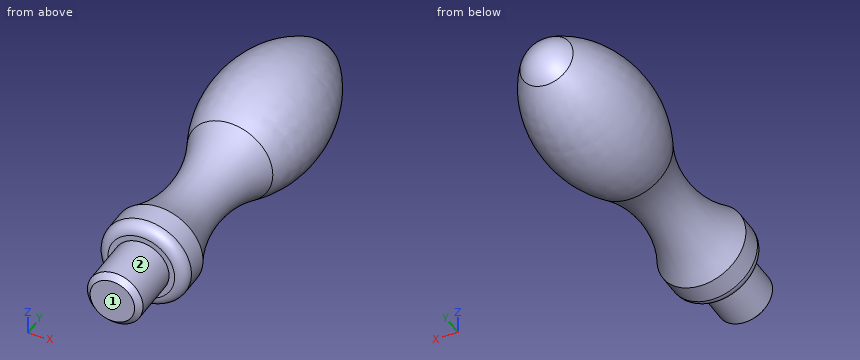
from build123d import *


with BuildPart() as part:
    # Sketch1 → Revolve1 (revolve)
    with BuildSketch(Plane.XY):
        with BuildLine():
            Line((0, 0), (4, 0))
            Line((4, 0), (5, 1))
            Line((5, 1), (5, 10))
            Line((5, 10), (6, 10))
            ThreePointArc((6, 10), (7.414213562, 10.585786438), (8, 12))
            Line((8, 12), (8, 16))
            ThreePointArc((8, 16), (5, 28.303061069), (7.726981853, 40.669502823))
            ThreePointArc((7.726981853, 40.669502823), (10.3121962, 55.557059673), (4.784815021, 69.620158175))
            ThreePointArc((4.784815021, 69.620158175), (2.671989048, 71.372194573), (0, 72))
            Line((0, 72), (0, 0))
        make_face()
    revolve(axis=Axis((0, -4.536906655, 0), (0, 1, 0)))


solid = part.part
Input: part model. Units: mm. Frame: model coordinates. Face numbers are marked on the shaded views. A direction names the side the tool comes from. Round coordinates to 2 decimals unless told otherwise and drop trailing zeros. Loops run counter-clockwise (first coordinate to the right, second up) from the corner with the lowest first, then second, coordinate; pieces in that order, holes last. Notation, with made-up numbers: M -35.5,-20.75 L -24.5,-20.75 A26 cw -24.5,-4.75 Z; hole C 28.25,27.5 d7. An arc over 180 degrees is marked long. Answer as CSV lines item,"result". Start each with the question number.
(1) Reachability of the marked faces 1 and 2 from +Z, -Z, +X, -X, +Y, -Y: full face, straight path, thin tool, end or side. Return the list, or none.
(2) Line query: line 1 (X direction, y = 11, z = 5.25); line 2 (X direction, y = 58, z = 4.75); line 3 (Z direction, x = -8.75, y = 46.5). Output: solid intervals per line, ascending. Write a range as [from, to].
(3) Section A-A, the plane y = 29. Output: boundary loops of the cut face in (x, z).
(4) First-contact query: pin 1 (2 mm diameter, centred on x = 4.5, y = 30, fed in from -Z); pin 2 (10 mm diameter, centred on y = 36.5, z = 2, fed in from +X); pin 3 (8 mm diameter, centred on y = 46, z = 6.5, fed in from -X). Flat tips, straight axial feed; report the tip coordinate or a pass-through.
Values found:
1,face 1,"+Z, -Z, +X, -X, -Y"
1,face 2,"-Y"
2,line 1,"x = [-5.68, 5.68]"
2,line 2,"x = [-8.75, 8.75]"
2,line 3,"z = [-4.31, 4.31]"
3,outline,"C 0,0 d10"
4,pin 1,"stops at z = -3.62"
4,pin 2,"stops at x = 8"
4,pin 3,"stops at x = -9.58"
